```python
from build123d import *

# Parameters (mm, degrees)
F0_W     = 15
F0_H     = 61
F0_W_2   = 12
F0_H_2   = 58
F1_DEPTH = 5
F2_W     = 17.5
F2_H     = 2.5
F2_W_2   = 11.5
F3_DEPTH = 3
F4_R     = 1
F5_W     = 4
F5_H     = 1
F6_DEPTH = 1
F7_R     = 0.49999
F8_W     = 4
F8_H     = 1
F9_DEPTH = 1
F10_R    = 0.49999


# Not quite as in the source:
# - a fillet or chamfer is up to 0.001 mm smaller than in the source, because OpenCascade refuses the exact size


with BuildPart() as f1:
    # F0 (on Top) → F1 (new body)
    with BuildSketch(Plane.XY):
        with Locations((-39.8457739502, 26.8311633799)):
            Rectangle(F0_W, F0_H)
        with Locations((-39.8457739502, 26.8311633799)):
            Rectangle(F0_W_2, F0_H_2, mode=Mode.SUBTRACT)
    extrude(amount=F1_DEPTH)

    # F2 (on face) → F3 (join)
    with BuildSketch(Plane.XY.offset(5)):
        with Locations((-31.0957739502, 57.0811633799)):
            Rectangle(F2_W, F2_H)
        with Locations((-48.5957739502, 57.0811633799)):
            Rectangle(F2_W, F2_H)
        with Locations((-31.0957739502, -3.4188366201)):
            Rectangle(F2_W, F2_H)
        with Locations((-48.5957739502, -3.4188366201)):
            Rectangle(F2_W, F2_H)
        with Locations((-28.0957739502, 35.0811633799)):
            Rectangle(F2_W_2, F2_H)
        with Locations((-28.0957739502, 18.5811633799)):
            Rectangle(F2_W_2, F2_H)
        with Locations((-51.5957739502, 18.5811633799)):
            Rectangle(F2_W_2, F2_H)
        with Locations((-51.5957739502, 35.0811633799)):
            Rectangle(F2_W_2, F2_H)
        with Locations((-28.0957739502, 46.5811633799)):
            Rectangle(F2_W_2, F2_H)
        with Locations((-28.0957739502, 7.0811633799)):
            Rectangle(F2_W_2, F2_H)
        with Locations((-51.5957739502, 46.5811633799)):
            Rectangle(F2_W_2, F2_H)
        with Locations((-51.5957739502, 7.0811633799)):
            Rectangle(F2_W_2, F2_H)
    extrude(amount=F3_DEPTH)

    # F4
    f4_edges = [f1.edges().sort_by_distance(p)[0] for p in [
        (-22.345774, 55.831163, 6.5),
        (-22.345774, 58.331163, 6.5),
        (-22.345774, 57.081163, 5),
        (-22.345774, 57.081163, 8),
        (-22.345774, 45.331163, 6.5),
        (-22.345774, 47.831163, 6.5),
        (-22.345774, 46.581163, 5),
        (-22.345774, 46.581163, 8),
        (-22.345774, 33.831163, 6.5),
        (-22.345774, 36.331163, 6.5),
        (-22.345774, 35.081163, 5),
        (-22.345774, 35.081163, 8),
        (-22.345774, 17.331163, 6.5),
        (-22.345774, 19.831163, 6.5),
        (-22.345774, 18.581163, 5),
        (-22.345774, 18.581163, 8),
        (-22.345774, 5.831163, 6.5),
        (-22.345774, 8.331163, 6.5),
        (-22.345774, 7.081163, 5),
        (-22.345774, 7.081163, 8),
        (-22.345774, -4.668837, 6.5),
        (-22.345774, -2.168837, 6.5),
        (-22.345774, -3.418837, 5),
        (-22.345774, -3.418837, 8),
        (-45.845774, 46.581163, 8),
        (-45.845774, 35.081163, 8),
        (-45.845774, 18.581163, 8),
        (-45.845774, 7.081163, 8),
        (-57.345774, -2.168837, 6.5),
        (-57.345774, -4.668837, 6.5),
        (-57.345774, -3.418837, 5),
        (-57.345774, -3.418837, 8),
        (-57.345774, 8.331163, 6.5),
        (-57.345774, 5.831163, 6.5),
        (-57.345774, 7.081163, 5),
        (-57.345774, 7.081163, 8),
        (-57.345774, 19.831163, 6.5),
        (-57.345774, 17.331163, 6.5),
        (-57.345774, 18.581163, 5),
        (-57.345774, 18.581163, 8),
        (-57.345774, 36.331163, 6.5),
        (-57.345774, 33.831163, 6.5),
        (-57.345774, 35.081163, 5),
        (-57.345774, 35.081163, 8),
        (-57.345774, 47.831163, 6.5),
        (-57.345774, 45.331163, 6.5),
        (-57.345774, 46.581163, 5),
        (-57.345774, 46.581163, 8),
        (-57.345774, 58.331163, 6.5),
        (-57.345774, 55.831163, 6.5),
        (-57.345774, 57.081163, 5),
        (-57.345774, 57.081163, 8),
        (-33.845774, 46.581163, 8),
        (-33.845774, 35.081163, 8),
        (-33.845774, 18.581163, 8),
        (-33.845774, 7.081163, 8),
        (-39.845774, 55.831163, 8),
        (-51.595774, 45.331163, 8),
        (-28.095774, 45.331163, 8),
        (-51.595774, 33.831163, 8),
        (-28.095774, 33.831163, 8),
        (-51.595774, 17.331163, 8),
        (-28.095774, 17.331163, 8),
        (-51.595774, 5.831163, 8),
        (-28.095774, 5.831163, 8),
        (-39.845774, -4.668837, 8),
        (-39.845774, -2.168837, 8),
        (-51.595774, 8.331163, 8),
        (-28.095774, 8.331163, 8),
        (-28.095774, 19.831163, 8),
        (-51.595774, 19.831163, 8),
        (-51.595774, 36.331163, 8),
        (-28.095774, 36.331163, 8),
        (-51.595774, 47.831163, 8),
        (-28.095774, 47.831163, 8),
        (-39.845774, 58.331163, 8),
    ]]
    fillet(f4_edges, radius=F4_R)

    # F5 (on face) → F6 (join)
    with BuildSketch(Plane.YZ.offset(-32.3457739502)):
        with Locations((26.8311633799, 1)):
            Rectangle(F5_W, F5_H)
    extrude(amount=F6_DEPTH)

    # F7 (radius 0.5 in the source; OpenCascade refuses exactly that, so slightly less here)
    f7_edges = [f1.edges().sort_by_distance(p)[0] for p in [
        (-31.345774, 26.831163, 1.5),
        (-31.345774, 24.831163, 1),
        (-31.345774, 26.831163, 0.5),
        (-31.345774, 28.831163, 1),
    ]]
    fillet(f7_edges, radius=F7_R)

    # F8 (on face) → F9 (join)
    with BuildSketch(Plane(origin=(-47.3457739502, 0, 0), x_dir=(0, -1, 0), z_dir=(-1, 0, 0))):
        with Locations((-26.8311633799, 1)):
            Rectangle(F8_W, F8_H)
    extrude(amount=F9_DEPTH)

    # F10 (radius 0.5 in the source; OpenCascade refuses exactly that, so slightly less here)
    f10_edges = [f1.edges().sort_by_distance(p)[0] for p in [
        (-48.345774, 26.831163, 1.5),
        (-48.345774, 28.831163, 1),
        (-48.345774, 26.831163, 0.5),
        (-48.345774, 24.831163, 1),
    ]]
    fillet(f10_edges, radius=F10_R)


solid = f1.part
```
Can you work these out from the model? Positions are in its coordinate system, mm. A direction names the side the tool comes from. Round coordinates to 2 decimals unless told otherwise and drop trailing zeros. Loops run counter-clockwise (first coordinate to the right, second up) from the corner with the lowest first, then second, coordinate; pieces in that order, holes last. Notation, with made-up numbers: (-23, 12) -> (23, 12) arc R20 cw to (23, 27) -> close; hole circle Ø7 at (49, 3.25). An arc over 180 degrees is marked (long way). One line per item, written item: value. Start each with the question number.
1. If we section it at C-C, the plane z = 3: Write out the boundary of the cut face in (x, y), then the cut area to 3 significant figures.
2. If we mould it in two halves opening along Y, with no side actions, what happens to faces 1 (the flat face through (-32.346, 26, 2)), 2 (the flat face through (-51, 5.831, 6)), 3 (the flat face through (-33, 41, 5)), 4 (the flat face through (-40, 57.331, 2))? For each: pulls with the +Y half, pulls with the -Y half, needs draft (parallel to the pull), parting line crosses it, or undercut.
3. For pin 1 (1.2 mm diameter, centred on x = -51.5, y = 35.5, fed in from -Z); pin 2 (3 mm diameter, centred on x = -53.5, y = 17, fed in from +Z); pin 3 (1.5 mm diameter, centred on x = -42, z = 3.5, fed in from +Y); pin 4 (1.6 mm diameter, centred on x = -33, y = 52.5, fed in from +Z), each with a flat end and sliding along its axis, tell me the tip position at first contact or that it passes through.
4. If we section it at D-D, the plane x = -25: Give the number of separate pieces and of enclosed holes in the cut face, then the cut area to 3 significant figures.
5. For faces 5 (the flat face through (-28, 47, 5)), 6 (the flat face through (-40, -4.669, 6)), 7 (the flat face through (-33, 2, 5)), which set-ups out of +Z, -Z, +X, -X, +Y, -Y let a thin tool reach every point of the face, with its end or its side?
6. If we section it at A-A, the plane y = 39: Write out the boundary of the cut face in (x, z), then the cut area to 3 significant figures.
7. If we section it at B-B, the plane x = -37.5: Write out the boundary of the cut face in (y, z), then the cut area to 3 significant figures.
8. If I drill on probe 1 along Y at (x, z) = (-41, 6.75); probe 2 along X at (y, z) = (45.5, 3.25); probe 3 along Y at (x, z) = (-36.5, 3.25), over which ranges is the centre line in solid material (lowest first)?
Calculated:
1. outline: (-47.35, -3.67) -> (-32.35, -3.67) -> (-32.35, 57.33) -> (-47.35, 57.33) -> close; hole (-45.85, -2.17) -> (-33.85, -2.17) -> (-33.85, 55.83) -> (-45.85, 55.83) -> close
1. area: 219 mm²
2. face 1: needs draft
2. face 2: undercut
2. face 3: undercut
2. face 4: pulls with the +Y half
3. pin 1: stops at z = 5
3. pin 2: stops at z = 8
3. pin 3: stops at y = 57.33
3. pin 4: stops at z = 5
4. separate pieces: 6
4. enclosed holes: 0
4. area: 42.4 mm²
5. face 5: -Z, +X, +Y, -Y
5. face 6: +Z, -Z, +X, -X, -Y
5. face 7: +Z, +X, -X
6. outline: (-47.35, 0) -> (-45.85, 0) -> (-45.85, 5) -> (-47.35, 5) -> close; (-33.85, 0) -> (-32.35, 0) -> (-32.35, 5) -> (-33.85, 5) -> close
6. area: 15.0 mm²
7. outline: (-4.67, 5) -> (-3.67, 5) -> (-3.67, 0) -> (-2.17, 0) -> (-2.17, 7) arc R1 ccw to (-3.17, 8) -> (-3.67, 8) arc R1 ccw to (-4.67, 7) -> close; (55.83, 0) -> (57.33, 0) -> (57.33, 5) -> (58.33, 5) -> (58.33, 7) arc R1 ccw to (57.33, 8) -> (56.83, 8) arc R1 ccw to (55.83, 7) -> close
7. area: 29.1 mm²
8. probe 1: y = -4.67 to -2.17, 55.83 to 58.33
8. probe 2: x = -47.35 to -45.85, -33.85 to -32.35
8. probe 3: y = -3.67 to -2.17, 55.83 to 57.33
